Source: CAD feature listing. Evaluate the final solid. Frame: model axes, mm. Face numbers are marked on the shaded views. Coordinates: 2 decimals unless noted, no trailing zeros. Loops run counter-clockwise (first coordinate to the right, second up) from the corner with the lowest first, then second, coordinate; pieces in that order, holes last. Notation, with made-up numbers: (37, 13.5) -> (75, 13.5) arc R19 ccw to (75, 47.5) -> close; hole circle Ø2 at (-7.5, 78). An arc over 180 degrees is marked (long way). Answer as a JSON object with one key per item and string values. Group by question number.
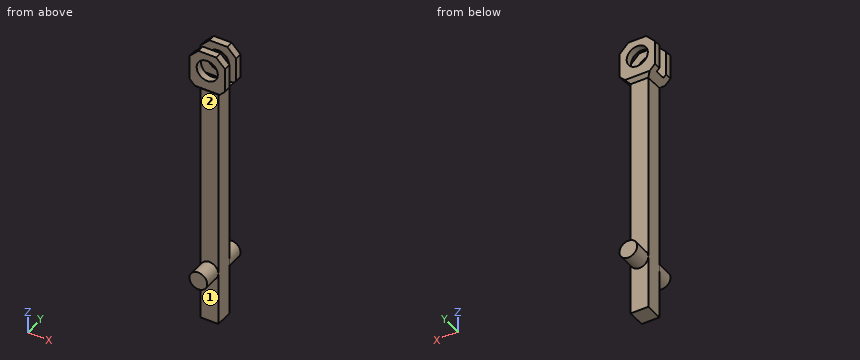
from build123d import *

# Parameters (mm, degrees)
SKETCH1_W                = 100
SKETCH1_H                = 100
BOSS_EXTRUDE1_DEPTH      = 1600
BOSS_EXTRUDE2_DEPTH      = 100
BOSS_EXTRUDE2_DEPTH_BACK = 200
SKETCH2_R                = 50
BOSS_EXTRUDE3_DEPTH      = 20
BOSS_EXTRUDE3_DEPTH_BACK = 120
SKETCH4_W                = 200
SKETCH4_H                = 234.974329415
CHAMFER1_SIZE            = 20
CHAMFER2_SIZE            = 50
SKETCH5_R                = 59.582841924
CUT_EXTRUDE2_DEPTH       = 560
SKETCH6_W                = 449.686922891
SKETCH6_H                = 60
CUT_EXTRUDE3_DEPTH       = 200


with BuildPart() as part:
    # Sketch1 → Boss-Extrude1 (new body)
    with BuildSketch(Plane.XY):
        with Locations((50, -50)):
            Rectangle(SKETCH1_W, SKETCH1_H)
    extrude(amount=BOSS_EXTRUDE1_DEPTH)

    # Sketch2 → Boss-Extrude2 (add, two sides: drawn at the far end of the back side and taken through both)
    with BuildSketch(Plane.XZ.offset(100).offset(-BOSS_EXTRUDE2_DEPTH_BACK)):
        with Locations(Location((50, 300, 0), (0, 0, 270))):
            Circle(SKETCH2_R)
    extrude(amount=BOSS_EXTRUDE2_DEPTH + BOSS_EXTRUDE2_DEPTH_BACK)

    # Sketch4 → Boss-Extrude3 (add, two sides: drawn at the far end of the back side and taken through both)
    with BuildSketch(Plane(origin=(0, 0, 0), x_dir=(1, 0, 0), z_dir=(0, 1, 0)).offset(-BOSS_EXTRUDE3_DEPTH_BACK)):
        with Locations((50, -1482.512835293)):
            Rectangle(SKETCH4_W, SKETCH4_H)
    extrude(amount=BOSS_EXTRUDE3_DEPTH + BOSS_EXTRUDE3_DEPTH_BACK)

    # Chamfer1
    chamfer1_edges = [part.edges().sort_by_distance(p)[0] for p in [
        (50, -120, 1365.025670585),
        (50, 20, 1365.025670585),
    ]]
    chamfer(chamfer1_edges, length=CHAMFER1_SIZE - 0.0001)  # a hair under: the kernel refuses the full size

    # Chamfer2
    chamfer2_edges = [part.edges().sort_by_distance(p)[0] for p in [
        (150, -50, 1365.025670585),
        (-50, -50, 1365.025670585),
        (150, -50, 1600),
        (-50, -50, 1600),
    ]]
    chamfer(chamfer2_edges, length=CHAMFER2_SIZE - 0.0001)  # a hair under: the kernel refuses the full size

    # Sketch5 → Cut-Extrude2 (cut)
    with BuildSketch(Plane.XZ.offset(120)):
        with Locations(Location((50, 1500, 0), (0, 0, 270))):
            Circle(SKETCH5_R)
    extrude(amount=-CUT_EXTRUDE2_DEPTH, mode=Mode.SUBTRACT)

    # Sketch6 → Cut-Extrude3 (cut)
    with BuildSketch(Plane.XY.offset(1600)):
        with Locations((52.387718175, -50)):
            Rectangle(SKETCH6_W, SKETCH6_H)
    extrude(amount=-CUT_EXTRUDE3_DEPTH, mode=Mode.SUBTRACT)


solid = part.part
1. Section query D-D on z = 841. Return loops of the section in (x, y), then the cut area to 3 significant figures.
2. Mould query, pull axis Z, two halves, no side actions, for the marked faces 1 and 2. Classes: pulls with the +Z half, pulls with the -Z half, needs draft (parallel to the pull), parting line crosses it, or undercut.
3. Ray query, L1, parallel to X at y = -7, z = 1500; L2, parallel to Y at x = -40, z = 1424.5; L3, parallel to Y at x = 12, z = 493. Return the intervals inside material, ascending.
4. Section query B-B on z = 1500. Return loops of the section in (x, y).
5. Pin query (flat end, axial travel): pin 1 Ø1 at (x, y) = (130, -109) entering from +Z; pin 2 Ø3 at (x, y) = (30.5, 36.5) entering from -Z; pin 3 Ø8 at (x, z) = (13.5, 1269) entering from +Y. Return the tip coordinate at first contact, or that it passes through.
6. Section query A-A on x = 50. State how many separate pieces and enclosed holes the cut face has, then the cut area to 3 significant figures.
Solved:
{
 "1": {"outline": "(0, -100) -> (100, -100) -> (100, 0) -> (0, 0) -> close", "area": "10,000 mm^2"},
 "2": {"face 1": "needs draft", "face 2": "undercut"},
 "3": {"L1": "-50 to -9.58, 109.58 to 150", "L2": "-120 to -80, -20 to 20", "L3": "-100 to 0"},
 "4": {"outline": "(-50, -120) -> (-9.58, -120) -> (-9.58, -80) -> (-50, -80) -> close; (-50, -20) -> (-9.58, -20) -> (-9.58, 20) -> (-50, 20) -> close; (109.58, -120) -> (150, -120) -> (150, -80) -> (109.58, -80) -> close; (109.58, -20) -> (150, -20) -> (150, 20) -> (109.58, 20) -> close"},
 "5": {"pin 1": "z = 1570.5", "pin 2": "z = 253.35", "pin 3": "y = 0"},
 "6": {"separate pieces": "3", "enclosed holes": "0", "area": "167,000 mm^2"}
}
